For this review, take the finished solid that the model builds, in its own axes (mm). Coordinates: 2 decimals unless noted, no trailing zeros. Loops run counter-clockwise (first coordinate to the right, second up) from the corner with the lowest first, then second, coordinate; pieces in that order, holes last. Notation, with made-up numbers: M 45,-37.5 L 92,-37.5 A22 cw 92,-4.5 Z; hole C -5,-9 d11. An arc over 180 degrees is marked long. Answer as a JSON object with one key per item and string values. Group by question number.
Item 1: Add section B-B (y = 17.5). State the section outline as (x, z) points, then the cut area to 3 significant figures.
Item 2: Add section A-A (z = 6.25). State the section outline as (x, y) points.
Item 3: Insertion check: pin 1 (5 mm diameter, centred on x = 272, z = 6.5, fed in from +Y); pin 2 (5 mm diameter, centred on y = -12, z = 1, fed in from +X); pin 3 (3 mm diameter, centred on x = -271.5, z = 4.5, fed in from -Y); pin 4 (3 mm diameter, centred on y = -18.5, z = 1, fed in from -X). Each pin has a flat end and moves straight along its axis. Give the tip position at first contact, or say it passes through.
Item 4: Wall thickness on L1, parallel to Y at x = 270, z = 6.25; L2, parallel to X at y = 16.5, z = 5: over which ranges is each line inside the solid? List them lowest first. Write a range as from..to.
from build123d import *

# Parameters (mm, degrees)
SKETCH1_W             = 550
SKETCH1_H             = 48
EXTRUDE_361_DEPTH     = 10
CUT_EXTRUDE_622_REACH = 278.226
SKETCH2_W             = 10
SKETCH2_H             = 13
CUT_EXTRUDE_942_REACH = 278.226
SKETCH3_R             = 1.5


with BuildPart() as part:
    # Sketch1 → Extrude 361 (new body)
    with BuildSketch(Plane.XY):
        Rectangle(SKETCH1_W, SKETCH1_H)
    extrude(amount=EXTRUDE_361_DEPTH)

    # Sketch2 → Cut-Extrude 622 (cut, up to next)
    with BuildSketch(Plane.XY.offset(10), mode=Mode.PRIVATE) as cut_extrude_622_sk1:
        with Locations((-270, -17.5)):
            Rectangle(SKETCH2_W, SKETCH2_H)
    cut_extrude_622_tool1 = extrude(cut_extrude_622_sk1.sketch, amount=-CUT_EXTRUDE_622_REACH, mode=Mode.PRIVATE) & part.part
    # Sketch2 → Cut-Extrude 622 (cut, up to next)
    with BuildSketch(Plane.XY.offset(10), mode=Mode.PRIVATE) as cut_extrude_622_sk2:
        with Locations((-270, 17.5)):
            Rectangle(SKETCH2_W, SKETCH2_H)
    cut_extrude_622_tool2 = extrude(cut_extrude_622_sk2.sketch, amount=-CUT_EXTRUDE_622_REACH, mode=Mode.PRIVATE) & part.part
    cut_extrude_622_1 = cut_extrude_622_tool1.solids().sort_by_distance((-270, -17.5, 10))[0]
    add(cut_extrude_622_1, mode=Mode.SUBTRACT)
    cut_extrude_622_2 = cut_extrude_622_tool2.solids().sort_by_distance((-270, 17.5, 10))[0]
    add(cut_extrude_622_2, mode=Mode.SUBTRACT)
    cut_extrude_622 = cut_extrude_622_1 + cut_extrude_622_2  # Cut-Extrude 622 as one shape, for the pattern or mirror that repeats it

    # Sketch3 → Cut-Extrude 942 (cut, up to next)
    with BuildSketch(Plane.XY.offset(10), mode=Mode.PRIVATE) as cut_extrude_942_sk1:
        with Locations((-270, 0)):
            Circle(SKETCH3_R)
    cut_extrude_942_tool1 = extrude(cut_extrude_942_sk1.sketch, amount=-CUT_EXTRUDE_942_REACH, mode=Mode.PRIVATE) & part.part
    cut_extrude_942 = cut_extrude_942_tool1.solids().sort_by_distance((-270, 0, 10))[0]
    add(cut_extrude_942, mode=Mode.SUBTRACT)

    # Mirror1: Cut-Extrude 622, Cut-Extrude 942 across plane
    add(cut_extrude_622.mirror(Plane(origin=(0, 0, 0), x_dir=(0, 0, 1), z_dir=(1, 0, 0))), mode=Mode.SUBTRACT)
    add(cut_extrude_942.mirror(Plane(origin=(0, 0, 0), x_dir=(0, 0, 1), z_dir=(1, 0, 0))), mode=Mode.SUBTRACT)


solid = part.part
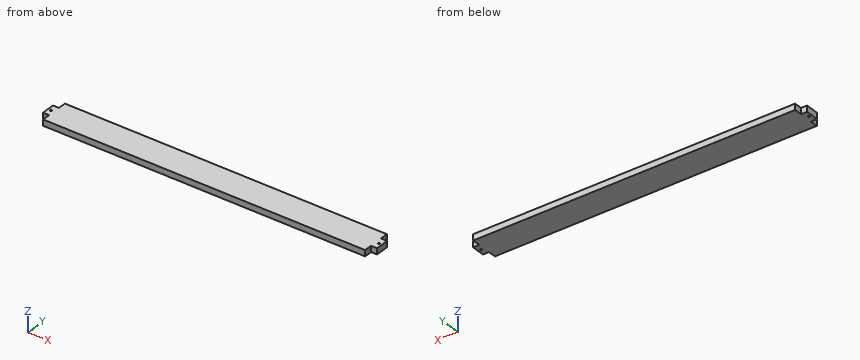
From the geometry:
{
 "1": {"outline": "M -265,0 L 265,0 L 265,10 L -265,10 Z", "area": "5,300 mm²"},
 "2": {"outline": "M -275,-11 L -265,-11 L -265,-24 L 265,-24 L 265,-11 L 275,-11 L 275,11 L 265,11 L 265,24 L -265,24 L -265,11 L -275,11 Z; hole C -270,0 d3; hole C 270,0 d3"},
 "3": {"pin 1": "stops at y = 11", "pin 2": "stops at x = 275", "pin 3": "stops at y = -11", "pin 4": "stops at x = -265"},
 "4": {"L1": "y = -11..-1.5, 1.5..11", "L2": "x = -265..265"}
}
